Read the model definition and answer for the solid it produces. Units are mm, in the model's axes. A direction names the side the tool comes from. Round coordinates to 2 decimals unless told otherwise and drop trailing zeros. Write each loop counter-clockwise with the first axis right and the second up, starting at its lowest first coordinate (ties: lowest second). Pieces come first, ordered by that corner, then holes.
from build123d import *

# Parameters (mm, degrees)
CHAMFER_1_SIZE = 1
FILLET_1_R     = 0.5
FILLET_2_R     = 0.25


with BuildPart() as part:
    # 草图2 → 旋转1 (revolve)
    with BuildSketch(Plane.XY, mode=Mode.PRIVATE) as revolve_1_sk:
        Polygon((0, 0), (0, 7.5), (6, 7.5), (6, 6), (56, 6), (60, 4.92820323), (60, 0), align=None)
    revolve(revolve_1_sk.sketch.rotate(Axis((-70.654432031, 0, 0), (1, 0, 0)), 90), axis=Axis((-70.654432031, 0, 0), (1, 0, 0)))

    # 倒角1
    chamfer_1_edges = [part.edges().sort_by_distance(p)[0] for p in [
        (6, 0, -7.5),
        (0, 0, -7.5),
    ]]
    chamfer(chamfer_1_edges, length=CHAMFER_1_SIZE)

    # 圆角1
    fillet_1_edges = [part.edges().sort_by_distance(p)[0] for p in [
        (6, 0, -6),
    ]]
    fillet(fillet_1_edges, radius=FILLET_1_R - 0.0001)  # a hair under: the kernel refuses the full size

    # 圆角2
    fillet_2_edges = [part.edges().sort_by_distance(p)[0] for p in [
        (60, 0, -4.92820323),
        (56, 0, -6),
    ]]
    fillet(fillet_2_edges, radius=FILLET_2_R)


solid = part.part
Q1. Section A-A (x = 9) is taken. Determine the outline of the cut face in (y, z), then the cut area to 3 significant figures.
Verdict:
outline: circle Ø12 at (0, 0)
area: 113 mm2
Q2. Straight lines are drawn through the part: probe 1 along Y at (x, z) = (33, -0.5); probe 2 along Z at (x, y) = (20, -0.75); probe 3 along Z at (x, y) = (51.5, -2.75). For each, find the intervals that lie inside material, in ascending order.
Verdict:
probe 1: y = -5.98 to 5.98
probe 2: z = -5.95 to 5.95
probe 3: z = -5.33 to 5.33
Q3. Flat-ended cylindrical pins translate along their axes: pin 1 Ø2 at (x, y) = (51.5, 5.5) entering from -Z; pin 2 Ø6 at (x, y) = (40, 4) entering from -Z; pin 3 Ø2 at (x, y) = (52.5, -1) entering from +Z. Find the tip coordinate at first contact, or state that the pin passes through.
Verdict:
pin 1: stops at z = -3.97
pin 2: stops at z = -5.92
pin 3: stops at z = 6
Q4. Which of the six approach directions +Z, -Z, +X, -X, +Y, -Y give full straight-line access (tool end or side, diameter ignored) to faces 1 (the cylindrical face through (3.028, -6.324, 4.032)), 2 (the cylindrical face through (31.58, 2.3, 5.54))?
Verdict:
face 1: +X, -X
face 2: +X
